from build123d import *

# Parameters (mm, degrees)
F1_DEPTH = 600
F2_R     = 0.5


with BuildPart() as f1:
    # F0 (on Front) → F1 (new body)
    with BuildSketch(Plane.XZ):
        Polygon((27.475, -40), (27.475, 40), (19.475, 40), (-27.475, 40), (-27.475, -40), align=None)
        Polygon((19.475, 40), (27.475, 40), (23.475, 45), align=None)
    extrude(amount=F1_DEPTH)

    # F2
    f2_edges = [f1.edges().sort_by_distance(p)[0] for p in [
        (23.475, -300, 45),
        (27.475, -300, 40),
        (19.475, -300, 40),
        (-27.475, -300, 40),
        (-27.475, -300, -40),
        (27.475, -300, -40),
    ]]
    fillet(f2_edges, radius=F2_R)


solid = f1.part
Design review of the part built by this model. Coordinates are the model's own, in mm. A direction names the side the tool comes from. Give positions to 0.01 mm unless a question says otherwise; leave off trailing zeros. Order: outer loops, then holes, each group sorted by start corner. A loop starts at its lowest first (then second) coordinate and runs counter-clockwise, first axis right, second up. Notation, with made-up numbers: (84, 25.25) - (98, 25.25) arc R12 ccw to (98, 35.25) - close; hole circle Ø3 at (-17.5, 29). An arc over 180 degrees is marked (long way). Use CSV: the item, a comma, the result in double quotes. Start each with the question number.
Q1. Take a section at A-A (y = -205). State the section outline as (x, z) points (3 decimals).
Q2. Machinability: for faces 1 (the face through (0, -296, -40)), 2 (the face through (-4, -296, 40)), which of the approach directions +Z, -Z, +X, -X, +Y, -Y give a long, thin tool a straight path to every point of the face, cutting with its end or side? Answer none if there is none.
Q3. For line 1 (Z direction, x = -21, y = -444.5); line 2 (Z direction, x = 25, y = -402.5); line 3 (X direction, y = -231, z = 41) (3 decimals), list the stretches that pass through material, from the lowest coordinate up.
Q4. For P1, Ø5, axis at x = 5, y = -230, coming from the +Z side; P2, Ø10, axis at x = -3, z = -15, coming from the +Y side, all flat-tipped, find the tip position at first contact; note any pin that passes through.
Q5. Take a section at B-B (x = 0.5). State the section outline as (y, z) points.
Calculated:
1,outline,"(-27.475, -39.5) arc R0.5 ccw to (-26.975, -40) - (26.975, -40) arc R0.5 ccw to (27.475, -39.5) - (27.475, 39.825) arc R0.5 ccw to (27.365, 40.137) - (23.865, 44.512) arc R0.5 ccw to (23.085, 44.512) - (19.625, 40.188) arc R0.5 cw to (19.235, 40) - (-26.975, 40) arc R0.5 ccw to (-27.475, 39.5) - close"
2,face 1,"-Z, +X, -X, +Y, -Y"
2,face 2,"+Z, -X, +Y, -Y"
3,line 1,"z = -40 to 40"
3,line 2,"z = -40 to 43.09"
3,line 3,"x = 20.275 to 26.675"
4,P1,"stops at z = 40"
4,P2,"stops at y = 0"
5,outline,"(-600, -40) - (0, -40) - (0, 40) - (-600, 40) - close"
